Source: three-view drawing plus pictorial views. Frame: mm from the lowest corner of the part. Give positions to 0.01 mm unless a question says otherwise; leave off trailing zeros. Loops run counter-clockwise (first coordinate to the right, second up) from the corner with the lowest first, then second, coordinate; pieces in that order, holes last. Notation, with made-up numbers: (-20.5, 74.25) - (12.5, 74.25) arc R21 ccw to (12.5, 86.25) - close; hole circle Ø4 at (64, -26.5). An arc over 180 degrees is marked (long way). Put each result on its own line as item: value.
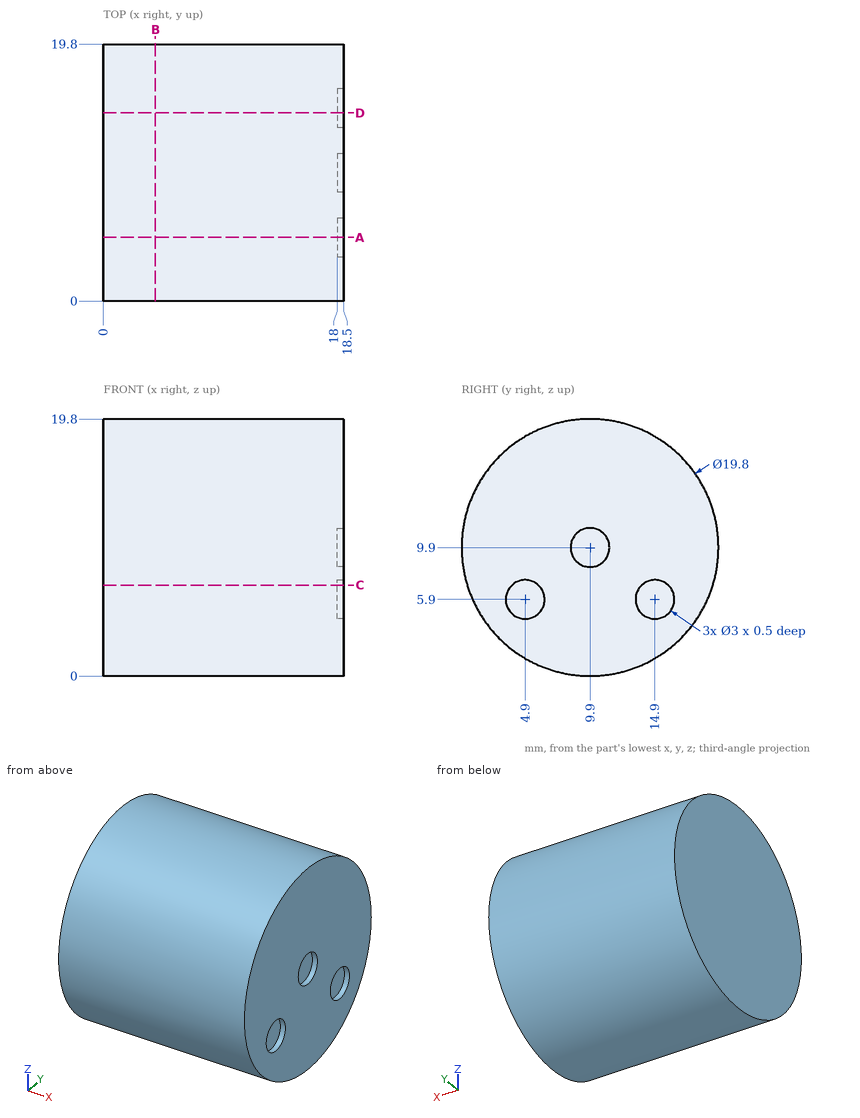
1) Section query B-B, the plane x = 4. Output: boundary loops of the cut face in (y, z).
Check result:
outline: circle Ø19.8 at (9.9, 9.9)
2) Section query A-A, the plane y = 4.9. Output: boundary loops of the cut face in (x, z), plus the area to 3 significant figures.
Check result:
outline: (0, 1.36) - (18.5, 1.36) - (18.5, 4.4) - (18, 4.4) - (18, 7.4) - (18.5, 7.4) - (18.5, 18.44) - (0, 18.44) - close
area: 315 mm²
3) Section query D-D, the plane y = 14.5. Output: boundary loops of the cut face in (x, z).
Check result:
outline: (0, 1.13) - (18.5, 1.13) - (18.5, 4.45) - (18, 4.45) - (18, 7.35) - (18.5, 7.35) - (18.5, 18.67) - (0, 18.67) - close
4) Section query C-C, the plane z = 7. Output: boundary loops of the cut face in (x, y).
Check result:
outline: (0, 0.43) - (18.5, 0.43) - (18.5, 3.88) - (18, 3.88) - (18, 5.92) - (18.5, 5.92) - (18.5, 13.88) - (18, 13.88) - (18, 15.92) - (18.5, 15.92) - (18.5, 19.37) - (0, 19.37) - close
5) Material intervals for line 1 along Y through (x, z) = (18.35, 5.9); line 2 along Y through (x, z) = (15, 17); line 3 along Y through (x, z) = (6.75, 14.5), sorted ascending. Write a range as [from, to].
Check result:
line 1: [0.84, 3.4], [6.4, 13.4], [16.4, 18.96]
line 2: [3, 16.8]
line 3: [1.13, 18.67]
6) Pin query (flat end, axial travel): P1, Ø2, axis at x = 3.5, z = 15, coming from the -Y side; P2, Ø0.9, axis at y = 9.5, z = 9.5, coming from the +X side; P3, Ø8, axis at x = 5.5, z = 16.5, coming from the +Y side. Return the tip coordinate at first contact, or that it passes through.
Check result:
P1: y = 0.89
P2: x = 18
P3: y = 19.45
